Autodesk Inventor part; units mm, degrees
ref_plane "YZ Plane" through (0, 0, 0) normal (1, 0, 0) x (0, 1, 0)
ref_plane "XZ Plane" through (0, 0, 0) normal (0, 1, 0) x (-1, 0, 0)
ref_plane "XY Plane" through (0, 0, 0) normal (0, 0, 1) x (1, 0, 0)
sketch "Sketch1" plane through (0, 0, 0) normal (0, 0, 1) x (1, 0, 0)
  line L0 (0, 0) -> (3, 0)
  line L1 (3, 0) -> (3, 72)
  line L2 (3, 72) -> (47, 72)
  line L3 (47, 72) -> (47, 0)
  line L4 (47, 0) -> (50, 0)
  line L5 (50, 0) -> (50, 75)
  line L6 (50, 75) -> (0, 75)
  line L7 (0, 75) -> (0, 0)
  dimension "d0" = 75
  dimension "d2" = 3
  dimension "d3" = 3
  dimension "d4" = 3
  dimension "d21" = 50
extrude "Extrusion1" add sketch "Sketch1" along normal mid plane 40
fillet "Fillet1" radius 3 1 edges at (50, 75, 0)
fillet "Fillet2" radius 3 1 edges at (0, 75, 0)
fillet "Fillet3" radius 20 1 edges at (48.5, 0, 20)
fillet "Fillet4" radius 20 1 edges at (1.5, 0, 20)
fillet "Fillet5" radius 20 1 edges at (48.5, 0, -20)
fillet "Fillet6" radius 20 1 edges at (1.5, 0, -20)
sketch "Sketch2" plane through (50, 72, 20) normal (1, 0, 0) x (0, 0, -1)
  arc A0 (0, -52) -> (40, -52) centre (20, -52) ccw
  circle A1 centre (20, -52) radius 5
  point P0 (20, -72)
  dimension "d13" = 10
extrude "Extrusion2" cut sketch "Sketch2" against normal through all
sketch "Sketch3" plane through (47, 75, 20) normal (0, 1, 0) x (1, 0, 0)
  line L0 (-47, 20) -> (3, 20) construction
  line L1 (3, 25) -> (3, 15)
  circle A0 centre (-22, 20) radius 10
  dimension "d16" = 20
extrude "Extrusion3" cut sketch "Sketch3" against normal blind 10
fillet "Fillet7" radius 3 1 edges at (47, 72, 0)
fillet "Fillet8" radius 3 1 edges at (3, 72, 0)
properties part number "Part1dia7demaio" material "Steel, Carbon"
Here's how the part is built. I have some questions about the finished solid (model axes, mm). A direction names the side the tool comes from. Coordinates: 2 decimals unless noted, no trailing zeros. Write each loop counter-clockwise with the first axis right and the second up, starting at its lowest first coordinate (ties: lowest second). Pieces come first, ordered by that corner, then holes. Notation, with made-up numbers: (53.5, -10.75) -> (57.5, -10.75) arc R24 cw to (57.5, 13.25) -> close; hole circle Ø7 at (48, 33). An arc over 180 degrees is marked (long way). Use a Markdown table: item, result. Add a question column.
(1) If we section it at C-C, the plane z = 8: Write out the boundary of the cut face in (x, y), and give its area (3 significant figures).
(2) If we section it at A-A, the plane y = 29: Write out the boundary of the cut face in (x, z).
(3) If we section it at B-B, the plane x = 25: Write out the boundary of the cut face in (y, z).
(4) If we section it at D-D, the plane z = -17: Write out the boundary of the cut face in (x, y).
(5) Please list where these lines run through material, in increasing order: line 1 (X direction, y = 51.5, z = 0.5); line 2 (Z direction, x = 25, y = 73.95); line 3 (Y direction, x = 1.15, z = 0).
(6) We'd pull the mould along Z, two halves only. Please class faces 3 (the flat face through (30, 75, -9)), 4 (the cylindrical face through (1.52, 15.12, 1.08)), 5 (the cylindrical face through (34.54, 73.52, -3)), 6 (the cylindrical face through (1.521, 5.703, -13.986)): +Z half, -Z half, draft (parallel to the pull), parting line (faces both ways), or undercut.
(7) For faces 1 (the flat face through (3, 34, 0)), 2 (the cylindrical face through (48.521, 6.014, 14.297)), which set-ups out of +Z, -Z, +X, -X, +Y, -Y let a thin tool reach every point of the face, with its end or its side?
(8) I'm going to push flat-ended pins straight in: P1, Ø6, axis at x = 43.5, z = 6.5, coming from the -Y side; P2, Ø12, axis at x = 30, z = -12, coming from the -Y side. Where does each tip first touch, or does it pass through?
Outcome:
| question | item | result |
|---|---|---|
| 1 | outline | (0, 1.67) -> (3, 1.67) -> (3, 69) arc R3 cw to (6, 72) -> (19, 72) -> (19, 75) -> (3, 75) arc R3 ccw to (0, 72) -> close; (31, 72) -> (44, 72) arc R3 cw to (47, 69) -> (47, 1.67) -> (50, 1.67) -> (50, 72) arc R3 ccw to (47, 75) -> (31, 75) -> close |
| 1 | area | 536 mm^2 |
| 2 | outline | (0, -20) -> (3, -20) -> (3, 20) -> (0, 20) -> close; (47, -20) -> (50, -20) -> (50, 20) -> (47, 20) -> close |
| 3 | outline | (72, -20) -> (75, -20) -> (75, -10) -> (72, -10) -> close; (72, 10) -> (75, 10) -> (75, 20) -> (72, 20) -> close |
| 4 | outline | (0, 9.46) -> (3, 9.46) -> (3, 69) arc R3 cw to (6, 72) -> (44, 72) arc R3 cw to (47, 69) -> (47, 9.46) -> (50, 9.46) -> (50, 72) arc R3 ccw to (47, 75) -> (3, 75) arc R3 ccw to (0, 72) -> close |
| 5 | line 1 | x = 0 to 3, 47 to 50 |
| 5 | line 2 | z = -20 to -10, 10 to 20 |
| 5 | line 3 | y = 0 to 15, 25 to 74.36 |
| 6 | face 3 | draft |
| 6 | face 4 | undercut |
| 6 | face 5 | undercut |
| 6 | face 6 | -Z half |
| 7 | face 1 | +Z, -Z, -Y |
| 7 | face 2 | +Z, +X, -X, -Y |
| 8 | P1 | stops at y = 70.66 |
| 8 | P2 | stops at y = 72 |
